```python
from build123d import *

# Parameters (mm, degrees)
F0_R      = 1.5
F1_DEPTH  = 1.7
F2_W      = 11.8
F2_H      = 9.1
F2_W_2    = 2.7
F3_DEPTH  = 11.2
F4_R      = 3.25
F4_R_2    = 0.75
F5_DEPTH  = 5
F2_W_3    = 9.5
F2_H_2    = 12
F2_W_4    = 7
F6_DEPTH  = 10.5
F2_W_5    = 65.85
F2_H_3    = 2.54
F2_W_6    = 5
F2_H_4    = 45
F2_W_7    = 60.5
F7_DEPTH  = 10.8
F9_W      = 103.9
F9_H      = 61.9
F10_DEPTH = 2
F11_W     = 2.4829882507
F11_H     = 22.3256796598
F11_W_2   = 9.5090560305
F12_DEPTH = 8.5
F11_W_3   = 8.2931313664
F11_H_2   = 29.6949772164
F13_DEPTH = 10
F11_W_4   = 9.6561443061
F11_H_3   = 24.203886278
F14_DEPTH = 20
F15_DEPTH = 28
F11_W_5   = 41.9279932976
F11_H_4   = 15.5006516725
F16_DEPTH = 20
F11_W_6   = 13.1828933954
F11_H_5   = 5.0447173417
F11_W_7   = 10.5653479695
F11_H_6   = 4.9971267581
F11_W_8   = 7.5681805611
F11_H_7   = 46.4369145338
F17_DEPTH = 11
F20_DEPTH = 1.6
F22_DEPTH = 20


with BuildPart() as f1:
    # F0 (on Top) → F1 (new body)
    with BuildSketch(Plane.XY):
        Polygon((97.0912873745, 0), (0, 0), (0, -53.34), (98.3443260193, -53.34), (101.6, -49.8757660389), (101.6, -14.9831408635), (99.4149968028, -12.760464102), (99.4149968028, -2.54), align=None)
        with Locations((13.97, -50.8)):
            Circle(F0_R, mode=Mode.SUBTRACT)
        with Locations((66.04, -45.72)):
            Circle(F0_R, mode=Mode.SUBTRACT)
        with Locations((96.52, -50.8)):
            Circle(F0_R, mode=Mode.SUBTRACT)
        with Locations((15.24, -2.54)):
            Circle(F0_R, mode=Mode.SUBTRACT)
        with Locations((90.17, -2.54)):
            Circle(F0_R, mode=Mode.SUBTRACT)
    extrude(amount=F1_DEPTH)

    # F2 (on face) → F3 (join)
    with BuildSketch(Plane.XY.offset(1.7)):
        with Locations((5.9, -45.19)):
            Rectangle(F2_W, F2_H)
        with Locations((-1.35, -45.19)):
            Rectangle(F2_W_2, F2_H)
    extrude(amount=F3_DEPTH)

    # F4 (on face) → F5 (cut)
    with BuildSketch(Plane(origin=(-2.7, 0, 0), x_dir=(0, -1, 0), z_dir=(-1, 0, 0))):
        with Locations((45.19, 8)):
            Circle(F4_R)
        with Locations((45.19, 8)):
            Circle(F4_R_2, mode=Mode.SUBTRACT)
    extrude(amount=-F5_DEPTH, mode=Mode.SUBTRACT)

    # F2 (on face) → F6 (join)
    with BuildSketch(Plane.XY.offset(1.7)):
        with Locations((4.75, -15)):
            Rectangle(F2_W_3, F2_H_2)
        with Locations((-3.5, -15)):
            Rectangle(F2_W_4, F2_H_2)
    extrude(amount=F6_DEPTH)

    # F2 (on face) → F7 (join)
    with BuildSketch(Plane.XY.offset(1.7)):
        with Locations((54.625, -2.37)):
            Rectangle(F2_W_5, F2_H_3)
        with Locations((95, -23.64)):
            Rectangle(F2_W_6, F2_H_4)
        with Locations((62.05, -50.37)):
            Rectangle(F2_W_7, F2_H_3)
    extrude(amount=F7_DEPTH)

    # F9 (on offset) → F10 (join)
    with BuildSketch(Plane.XY.offset(12.5)):
        with Locations((51.42, -30.17)):
            Rectangle(F9_W, F9_H)
    extrude(amount=F10_DEPTH)

    # F11 (on face) → F12 (join)
    with BuildSketch(Plane.XY.offset(14.5)):
        with Locations((-1.7714941254, -47.3081059754)):
            Rectangle(F11_W, F11_H)
        with Locations((4.2245280153, -47.3081059754)):
            Rectangle(F11_W_2, F11_H)
    extrude(amount=F12_DEPTH)

    # F11 (on face) → F13 (join)
    with BuildSketch(Plane.XY.offset(14.5)):
        with Locations((12.792323716, -21.0819304921)):
            Rectangle(F11_W_3, F11_H_2)
    extrude(amount=F13_DEPTH)

    # F11 (on face) → F14 (join)
    with BuildSketch(Plane.XY.offset(14.5)):
        with Locations((23.1177126989, -18.6045370065)):
            Rectangle(F11_W_4, F11_H_3)
    extrude(amount=F14_DEPTH)

    # F11 (on face) → F15 (join)
    with BuildSketch(Plane.XY.offset(14.5)):
        Polygon((26.9871652126, -35.5093516409), (19.7103302926, -33.7288491428), (13.8745306454, -57.4684444644), (21.1770047413, -59.2552203791), align=None)
    extrude(amount=F15_DEPTH)

    # F11 (on face) → F16 (join)
    with BuildSketch(Plane.XY.offset(14.5)):
        Polygon((30.1127098501, -33.6817987263), (30.1127098501, -49.3730306625), (91.5435701609, -49.3730306625), (91.5435701609, -33.6817987263), (86.4100605249, -33.6817987263), (76.222717762, -33.6817987263), align=None)
        with Locations((50.3709092736, -18.5092454776)):
            Rectangle(F11_W_5, F11_H_4)
    extrude(amount=F16_DEPTH)

    # F11 (on face) → F17 (join)
    with BuildSketch(Plane.XY.offset(14.5)):
        with Locations((78.7578299642, -56.7604172975)):
            Rectangle(F11_W_6, F11_H_5)
        with Locations((95.4863019288, -56.7842125893)):
            Rectangle(F11_W_7, F11_H_6)
        with Locations((96.6827124357, -23.6736045626)):
            Rectangle(F11_W_8, F11_H_7)
    extrude(amount=F17_DEPTH)

    # F19 (on offset) → F20 (join)
    with BuildSketch(Plane.XY.offset(25.5)):
        Polygon((92.734746635, -50.1511096954), (89.1940370202, -53.6969974637), (71.7452839017, -53.6969974637), (68.7820387674, -56.720264256), (68.7820387674, -68.3501685575), (71.7745572329, -71.3383169692), (85.3640451386, -71.3383169692), (88.3478298783, -68.3501685575), (103.9278417004, -68.3501685575), (107.1784873109, -65.094769001), (107.1784873109, -62.4223748591), (108.7936833501, -60.804816657), (110.7314362108, -60.804816657), (115.7298460603, -55.7990968227), (115.7298460603, -17.3471495509), (110.9337881207, -12.3451392372), (108.7346714968, -12.3451392372), (105.7346100416, -9.3494588509), (105.7346100416, -3.3496673639), (102.7355343103, -0.3549712621), (95.7330679293, -0.3549712621), (92.734746635, -3.3576774877), align=None)
    extrude(amount=F20_DEPTH)

    # F21 (on face) → F22 (join)
    with BuildSketch(Plane.XY.offset(27.1)):
        Polygon((113.4268465994, -14.9452546611), (114.0775308013, -15.6238805514), (114.0775308013, -14.9452546611), align=None)
        Polygon((105.269394815, -14.9452546611), (105.269394815, -35.3506803513), (114.0775308013, -35.3506803513), (114.0775308013, -15.6238805514), (113.4268465994, -14.9452546611), align=None)
        Polygon((114.0775308013, -58.2013837993), (114.0775308013, -57.4538285301), (113.3310672068, -58.2013837993), align=None)
        Polygon((113.3310672068, -58.2013837993), (114.0775308013, -57.4538285301), (114.0775308013, -37.8092862666), (105.269394815, -37.8092862666), (105.269394815, -58.2013837993), align=None)
    extrude(amount=F22_DEPTH)


solid = f1.part
```
Can you work these out from the model? Positions are in its coordinate system, mm. A direction names the side the tool comes from. Coordinates: 2 decimals unless noted, no trailing zeros. Loops run counter-clockwise (first coordinate to the right, second up) from the corner with the lowest first, then second, coordinate; pieces in that order, holes last. Notation, with made-up numbers: (-3.5, 18) - (1.5, 18) arc R14 cw to (1.5, 31) - close; hole circle Ø1 at (83, -34.75). An arc over 180 degrees is marked (long way). Answer as CSV lines item,"result". Start each with the question number.
1) I need wall thicknesses on line 1 (Z direction, x = -1, y = -45); line 2 (X direction, y = -29, z = 22.5); line 3 (X direction, y = -21, z = 29.5). Which ranges of each line are inside material? Lowest first, please. Write a range as from..to.
2) Which directions (+Z, -Z, +X, -X, +Y, -Y) give clear straight access to the entire face, cutting with the end or side of a thin tool? Please do faces 4 (the flat face through (79, -54.238, 20)), 5 (the cylindrical face through (12.86, -49.79, 0.84)), 6 (the flat face through (92.5, -24, 7)), 7 (the flat face through (70.28, -55.19, 26.29)), 8 (the flat face through (13, -6.234, 19)).
3) Thinking about a two-plate mould opening in Z: for faces 1 (the flat face through (31.8, -50, 7)), 2 (the flat face through (-1, -45, 1.7)), 3 (the flat face through (61, -33.682, 24)), which applies, pulls with the +Z half, pulls with the -Z half, needs draft (parallel to the pull), parting line crosses it, or undercut?
4) Suppose I cut it at A-A (x = 56.5). Please give me the cut outline in (y, z).
5) For pin 1 (5.5 mm diameter, centred on y = -56, z = 20, fed in from -X); pin 2 (0.5 mm diameter, centred on y = -35.5, z = 26, fed in from -X); pin 3 (2 mm diameter, centred on y = -33.5, z = 15, fed in from +X), each with a flat end and sliding along its axis, tell me the tip position at first contact or that it passes through.
Check result:
1,line 1,"z = 1.7..4.76, 7.27..8.73, 11.24..12.9, 14.5..23"
1,line 2,"x = 8.65..16.94, 18.29..27.95, 92.9..100.47"
1,line 3,"x = 18.29..27.95, 29.41..71.33, 105.27..114.08"
2,face 4,"+X"
2,face 5,"-Z"
2,face 6,"+Y, -Y"
2,face 7,"+Z"
2,face 8,"+Z, -X, +Y"
3,face 1,"undercut"
3,face 2,"pulls with the -Z half"
3,face 3,"needs draft"
4,outline,"(-61.12, 12.5) - (-51.64, 12.5) - (-51.64, 1.7) - (-53.34, 1.7) - (-53.34, 0) - (0, 0) - (0, 1.7) - (-1.1, 1.7) - (-1.1, 12.5) - (0.78, 12.5) - (0.78, 14.5) - (-10.76, 14.5) - (-10.76, 34.5) - (-26.26, 34.5) - (-26.26, 14.5) - (-33.68, 14.5) - (-33.68, 34.5) - (-49.37, 34.5) - (-49.37, 14.5) - (-61.12, 14.5) - close; hole (-49.1, 1.7) - (-3.64, 1.7) - (-3.64, 12.5) - (-49.1, 12.5) - close"
5,pin 1,"stops at x = -3.01"
5,pin 2,"stops at x = 19.21"
5,pin 3,"stops at x = 103.37"
